Geometry check sheet. Reference: the model listing, model coordinates, mm. Face numbers are marked on the shaded views. A direction names the side the tool comes from. Round coordinates to 2 decimals unless told otherwise and drop trailing zeros. Write each loop counter-clockwise with the first axis right and the second up, starting at its lowest first coordinate (ties: lowest second). Pieces come first, ordered by that corner, then holes.
Item 1: Draft check along X on the marked faces 6, 7, 8 and 9. Enter one of: pulls with the +X half, pulls with the -X half, needs draft (parallel to the pull), parting line crosses it, or undercut.
Item 2: Cross-section at B-B (y = -13). Enter the section's corners in (x, z), then the cut area to 3 significant figures.
Item 3: Cross-section at D-D (z = -5). Enter the section's corners in (x, y).
Item 4: Access from +Z, -Z, +X, -X, +Y, -Y to the whole of each face (thin tool, end or side, straight path). Record for the marked faces 1, 2, 3, 4 and 5.
Item 5: Scan lines: probe 1 along X at (y, z) = (-16.5, 14); probe 2 along Z at (x, y) = (-15, -56.5); probe 3 along Z at (x, y) = (-3, -22). Record each from-to range of solid material in increasing order.
Item 6: Cross-section at C-C (x = -49.5). Enter the section's corners in (y, z), then the cut area to 3 significant figures.
Item 7: Cross-section at A-A (z = 31). Enter the section's corners in (x, y).
Item 8: Depth check by flat-ended pin: P1, Ø7.5, axis at y = -12, z = -13, coming from the +X side; P2, Ø10, axis at x = -29.5, y = -26, coming from the +Z side; P3, Ø21.5, axis at x = -41.5, y = -52.5, coming from the -Z side; P4, Ø20.5, axis at y = -19, z = 16, coming from the +X side. Enter the tip coordinate at first touch or a pass-through.
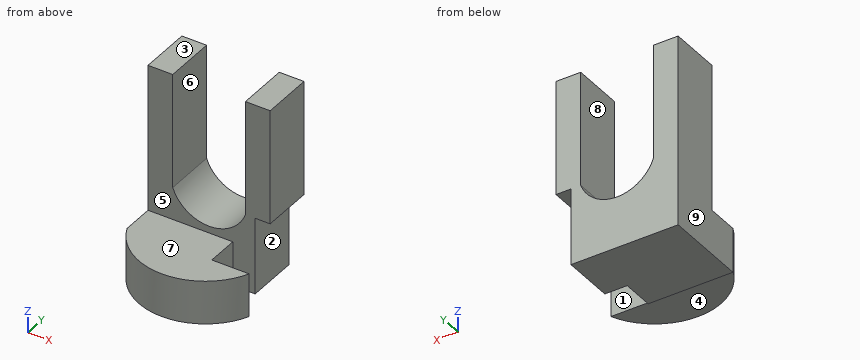
from build123d import *

# Parameters (mm, degrees)
F1_DEPTH = 25.4
F0_W     = 60.0766055286
F0_H     = 21.8948144466
F2_DEPTH = 41.148
F4_DEPTH = 21.336
F6_DEPTH = 7.366
F8_DEPTH = 21.8958144466


with BuildPart() as f1:
    # F0 (on Front) → F1 (new body)
    with BuildSketch(Plane.XZ):
        with BuildLine():
            Line((-47.9169413447, 56.5039552748), (-60.0766055286, 56.5039552748))
            Line((-60.0766055286, 56.5039552748), (-60.0766055286, -15.9127693623))
            Line((-60.0766055286, -15.9127693623), (0, -15.9127693623))
            Line((0, -15.9127693623), (0, 56.5039552748))
            Line((0, 56.5039552748), (-12.1596641839, 56.5039552748))
            Line((-12.1596641839, 56.5039552748), (-12.1596641839, 0))
            ThreePointArc((-12.1596641839, 0), (-30.0383027643, -12.5509662024), (-47.9169413447, 0))
            Line((-47.9169413447, 0), (-47.9169413447, 56.5039552748))
        make_face()
    extrude(amount=F1_DEPTH)

    # F0 (on Front) → F2 (join)
    with BuildSketch(Plane.XZ):
        with Locations((-30.0383027643, -26.8601765856)):
            Rectangle(F0_W, F0_H)
    extrude(amount=F2_DEPTH)

    # F3 (on face) → F4 (join)
    with BuildSketch(Plane.XY.offset(-15.9127693623)):
        with BuildLine():
            Line((0, -41.148), (-60.0766055286, -41.148))
            ThreePointArc((-60.0766055286, -41.148), (-30.0383027643, -60.8627597927), (0, -41.148))
        make_face()
    extrude(amount=-F4_DEPTH)

    # F5 (on face) → F6 (cut)
    with BuildSketch(Plane.YZ):
        Polygon((0, 0), (-25.4, 0), (-25.4, -15.9127693623), (-25.4, -37.8075838089), (0, -37.8075838089), align=None)
    extrude(amount=-F6_DEPTH, mode=Mode.SUBTRACT)

    # F7 (on face) → F8 (cut, through all)
    with BuildSketch(Plane.XY.offset(-15.9127693623)):
        Polygon((-7.366, -25.4), (-18.3683019131, -25.4), (-18.3683019131, -41.148), (0, -41.148), (0, -25.4), align=None)
    extrude(amount=-F8_DEPTH, mode=Mode.SUBTRACT)


solid = f1.part
Resolved:
1. face 6: undercut
1. face 7: needs draft
1. face 8: undercut
1. face 9: pulls with the -X half
2. outline: (-60.08, -37.81) - (-7.37, -37.81) - (-7.37, 0) - (0, 0) - (0, 56.5) - (-12.16, 56.5) - (-12.16, 0) arc R19.01 cw to (-47.92, 0) - (-47.92, 56.5) - (-60.08, 56.5) - close
2. area: 3,040 mm2
3. outline: (-60.08, -25.4) - (-45.21, -25.4) - (-45.21, 0) - (-60.08, 0) - close; (-14.87, -25.4) - (-7.37, -25.4) - (-7.37, 0) - (-14.87, 0) - close
4. face 1: +Z, -Z, +X
4. face 2: -Z, +X, +Y
4. face 3: +Z, +X, -X, +Y, -Y
4. face 4: -Z, +X, -X, -Y
4. face 5: +Z, +X
5. probe 1: x = -60.08 to -47.92, -12.16 to 0
5. probe 2: z = -37.25 to -15.91
5. probe 3: z = 0 to 56.5
6. outline: (-54.45, -37.25) - (-41.15, -37.25) - (-41.15, -37.81) - (0, -37.81) - (0, 56.5) - (-25.4, 56.5) - (-25.4, -15.91) - (-54.45, -15.91) - close
6. area: 3,020 mm2
7. outline: (-60.08, -25.4) - (-47.92, -25.4) - (-47.92, 0) - (-60.08, 0) - close; (-12.16, -25.4) - (0, -25.4) - (0, 0) - (-12.16, 0) - close
8. P1: stops at x = -7.37
8. P2: stops at z = -11.74
8. P3: stops at z = -37.25
8. P4: stops at x = 0
